Autodesk Inventor part; units mm, degrees
ref_plane "YZ Plane" through (0, 0, 0) normal (1, 0, 0) x (0, 1, 0)
ref_plane "XZ Plane" through (0, 0, 0) normal (0, 1, 0) x (-1, 0, 0)
ref_plane "XY Plane" through (0, 0, 0) normal (0, 0, 1) x (1, 0, 0)
sketch "Sketch1" plane through (0, 0, 0) normal (0, 0, 1) x (1, 0, 0)
  line L0 (8.0225, -1.3281) -> (-10.4075, -1.3281)
  line L1 (-10.4075, -1.3281) -> (-10.4075, 3.0719)
  line L2 (-10.4075, 3.0719) -> (8.0225, 3.0719)
  line L3 (8.0225, 3.0719) -> (8.0225, -1.3281)
  point P0 (0, 0)
  dimension "d0" = 18.43
  dimension "d1" = 4.4
extrude "Extrusion1" add sketch "Sketch1" along normal blind 2
sketch "Sketch2" plane through (-10.4075, 3.0719, 0) normal (0, 1, 0) x (1, 0, 0)
  line L0 (0, 0) -> (18.43, 0)
  line L1 (18.43, 0) -> (18.43, -2)
  line L2 (2.415, 0) -> (16.015, 0)
  line L3 (16.015, 0) -> (16.015, -1)
  line L4 (16.015, -1) -> (2.415, -1)
  line L5 (2.415, -1) -> (2.415, 0)
  point P0 (10.4075, 0)
  dimension "d4" = 13.6
  dimension "d5" = 2.415
  dimension "d6" = 0
  dimension "d7" = 1
extrude "Extrusion2" cut sketch "Sketch2" against normal blind 1
properties part number "FlatFlex26"
Geometry: final body of the model. Coordinates: model frame, mm. A direction names the side the tool comes from. Give positions to 0.01 mm unless a question says otherwise; leave off trailing zeros. Write each loop counter-clockwise with the first axis right and the second up, starting at its lowest first coordinate (ties: lowest second). Pieces come first, ordered by that corner, then holes. Notation, with made-up numbers: (18, 13.25) -> (60, 13.25) arc R31 ccw to (60, 48.25) -> close; hole circle Ø3 at (60.25, -20). An arc over 180 degrees is marked (long way). Answer in a Markdown table with one row per item.
(1) Section query B-B on x = -1.5. Return loops of the section in (y, z), then the cut area to 3 significant figures.
Answers below:
| item | result |
|---|---|
| outline | (-1.33, 0) -> (2.07, 0) -> (2.07, 1) -> (3.07, 1) -> (3.07, 2) -> (-1.33, 2) -> close |
| area | 7.80 mm^2 |
(2) Draft query along X for faces 1 (the flat face through (-1, 1, 2)), 2 (the flat face through (-10.408, 1, 1)), 3 (the flat face through (-1.1, 2.6, 1)). Return one class per face: +X half, -X half, draft (parallel to the pull), parting line (faces both ways), or undercut.
Answers below:
| item | result |
|---|---|
| face 1 | draft |
| face 2 | -X half |
| face 3 | undercut |
(3) Section query A-A on z = 0.5. Return loops of the section in (x, y).
Answers below:
| item | result |
|---|---|
| outline | (-10.41, -1.33) -> (8.02, -1.33) -> (8.02, 3.07) -> (5.61, 3.07) -> (5.61, 2.07) -> (-7.99, 2.07) -> (-7.99, 3.07) -> (-10.41, 3.07) -> close |
(4) Ray query, line 1 along X through (y, z) = (2.15, 0.75); line 2 along Y through (x, z) = (1, 0.3); line 3 along Z through (x, y) = (-7, 2.6). Return the intervals inside material, ascending. Write a range as [from, to].
Answers below:
| item | result |
|---|---|
| line 1 | [-10.41, -7.99], [5.61, 8.02] |
| line 2 | [-1.33, 2.07] |
| line 3 | [1, 2] |
(5) Pin query (flat end, axial travel): pin 1 (0.8 mm diameter, centred on x = -4.5, z = 0.5, fed in from +Y). Return the tip coordinate at first contact, or that it passes through.
Answers below:
| item | result |
|---|---|
| pin 1 | y = 2.07 |
(6) Set-up query: faces 4 (the flat face through (8.023, 1, 1)), 5 (the flat face through (-1.3, 2.072, 0.5)). Return all of +Z, -Z, +X, -X, +Y, -Y with unobstructed straight access to the full face (end or side cutting, diameter ignored); none if empty.
Answers below:
| item | result |
|---|---|
| face 4 | +Z, -Z, +X, +Y, -Y |
| face 5 | -Z, +Y |
(7) Section query C-C on y = 2.4. Return loops of the section in (x, z).
Answers below:
| item | result |
|---|---|
| outline | (-10.41, 0) -> (-7.99, 0) -> (-7.99, 1) -> (5.61, 1) -> (5.61, 0) -> (8.02, 0) -> (8.02, 2) -> (-10.41, 2) -> close |
